For this review, take the finished solid that the model builds, in its own axes (mm). Face numbers are marked on the shaded views. A direction names the side the tool comes from. Round coordinates to 2 decimals unless told otherwise and drop trailing zeros. Order: outer loops, then holes, each group sorted by start corner. A loop starts at its lowest first (then second) coordinate and runs counter-clockwise, first axis right, second up. Notation, with made-up numbers: M -22,14 L -7,14 A26 ccw -7,43 Z; hole C 49.5,66.5 d5. An arc over 180 degrees is marked long. Use a Markdown table: item, result.
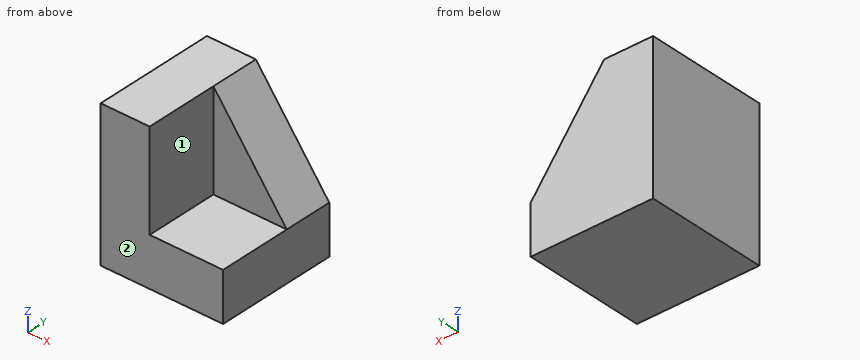
from build123d import *

# Parameters (mm, degrees)
F1_DEPTH = 50
F3_DEPTH = 20


with BuildPart() as f1:
    # F0 (on Front) → F1 (new body)
    with BuildSketch(Plane.XZ):
        Polygon((0, 60), (0, 0), (50, 0), (50, 20), (20, 20), (20, 60), align=None)
    extrude(amount=F1_DEPTH)

    # F2 (on face) → F3 (join)
    with BuildSketch(Plane(origin=(0, 0, 0), x_dir=(-1, 0, 0), z_dir=(0, 1, 0))):
        Polygon((-20, 20), (-20, 60), (-50, 20), align=None)
    extrude(amount=-F3_DEPTH)


solid = f1.part
Q1. Clearance check with a flat-ended pin moving along its axis: pin 1 (1 mm diameter, centred on x = 23, z = 27.5, fed in from -Y). State where the tip first meets the part, or that it passes through.
Determined:
| item | result |
|---|---|
| pin 1 | stops at y = -20 |
Q2. Add section C-C (y = -3.5). Write out the cut boundary in (x, z), then the cut area to 3 significant figures.
Determined:
| item | result |
|---|---|
| outline | M 0,0 L 50,0 L 50,20 L 20,60 L 0,60 Z |
| area | 2,400 mm^2 |
Q3. Add section B-B (z = 39). Write out the cut boundary in (x, y), then the cut area to 4 significant figures.
Determined:
| item | result |
|---|---|
| outline | M 0,-50 L 20,-50 L 20,-20 L 35.75,-20 L 35.75,0 L 0,0 Z |
| area | 1,315 mm^2 |
Q4. Machinability: for the marked faces 1 and 2, which of the approach directions +Z, -Z, +X, -X, +Y, -Y give a long, thin tool a straight path to every point of the face, cutting with its end or side? Answer none if there is none.
Determined:
| item | result |
|---|---|
| face 1 | +Z, +X, -Y |
| face 2 | +Z, -Z, +X, -X, -Y |
Q5. Wall thickness on line 1 along Y through (x, z) = (23.5, 37); line 2 along Z through (x, y) = (47, -21): over which ranges is each line inside the solid? List them lowest first. Write a range as [from, to].
Determined:
| item | result |
|---|---|
| line 1 | y = [-20, 0] |
| line 2 | z = [0, 20] |
Q6. Add section A-A (y = -28.5). Write out the cut boundary in (x, z), then the cut area to 3 significant figures.
Determined:
| item | result |
|---|---|
| outline | M 0,0 L 50,0 L 50,20 L 20,20 L 20,60 L 0,60 Z |
| area | 1,800 mm^2 |
